Verification items for this drawing (mm, ordinates from the low corner). Round coordinates to 2 decimals unless told otherwise and drop trailing zeros. Loops run counter-clockwise (first coordinate to the right, second up) from the corner with the lowest first, then second, coordinate; pieces in that order, holes last. Notation, with made-up numbers: (45.25, -33.75) -> (63.25, -33.75) arc R26 ccw to (63.25, -13.75) -> close; hole circle Ø11 at (-13, 56.25). An arc over 180 degrees is marked (long way). One line per question, with ' | ' between items.
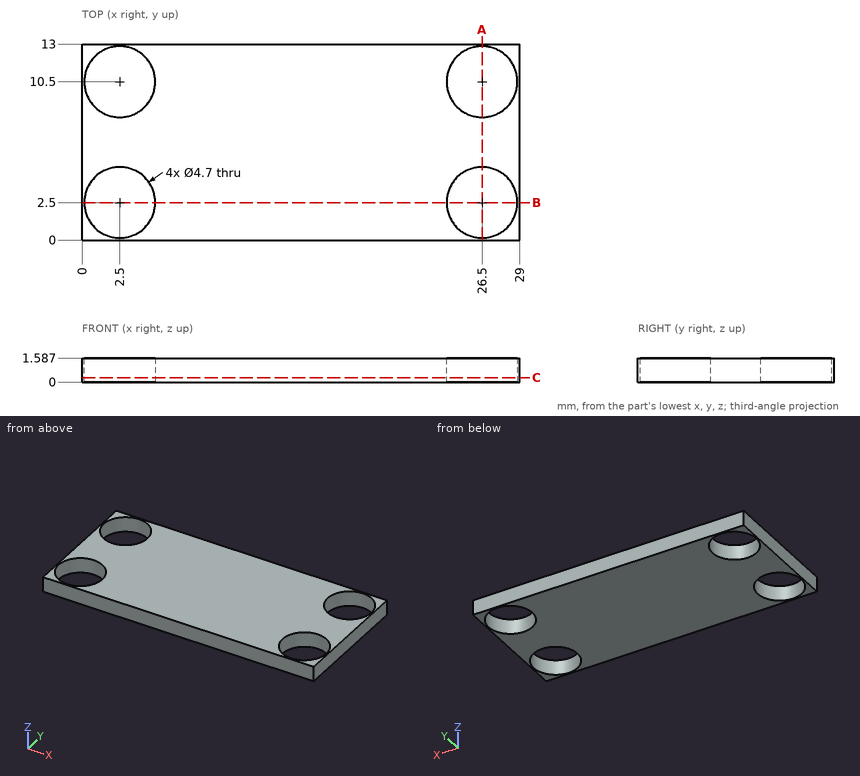
(1) Sectioned sample at B-B, the plane y = 2.5. Record the cut outline in (x, z).
Answer:
outline: (0, 0) -> (0.15, 0) -> (0.15, 1.59) -> (0, 1.59) -> close; (4.85, 0) -> (24.15, 0) -> (24.15, 1.59) -> (4.85, 1.59) -> close; (28.85, 0) -> (29, 0) -> (29, 1.59) -> (28.85, 1.59) -> close
(2) Scan lines: probe 1 along Y at (x, z) = (26.5, 1.2); probe 2 along Y at (x, z) = (27.75, 0.45); probe 3 along X at (y, z) = (1, 0.2). Record each from-to range of solid material in increasing order.
Answer:
probe 1: y = 0 to 0.15, 4.85 to 8.15, 12.85 to 13 | probe 2: y = 0 to 0.51, 4.49 to 8.51, 12.49 to 13 | probe 3: x = 0 to 0.69, 4.31 to 24.69, 28.31 to 29
(3) Sectioned sample at A-A, the plane x = 26.5. Record the cut outline in (y, z).
Answer:
outline: (0, 0) -> (0.15, 0) -> (0.15, 1.59) -> (0, 1.59) -> close; (4.85, 0) -> (8.15, 0) -> (8.15, 1.59) -> (4.85, 1.59) -> close; (12.85, 0) -> (13, 0) -> (13, 1.59) -> (12.85, 1.59) -> close
(4) Sectioned sample at C-C, the plane z = 0.3. Record the cut outline in (x, y).
Answer:
outline: (0, 0) -> (29, 0) -> (29, 13) -> (0, 13) -> close; hole circle Ø4.7 at (2.5, 2.5); hole circle Ø4.7 at (2.5, 10.5); hole circle Ø4.7 at (26.5, 2.5); hole circle Ø4.7 at (26.5, 10.5)
